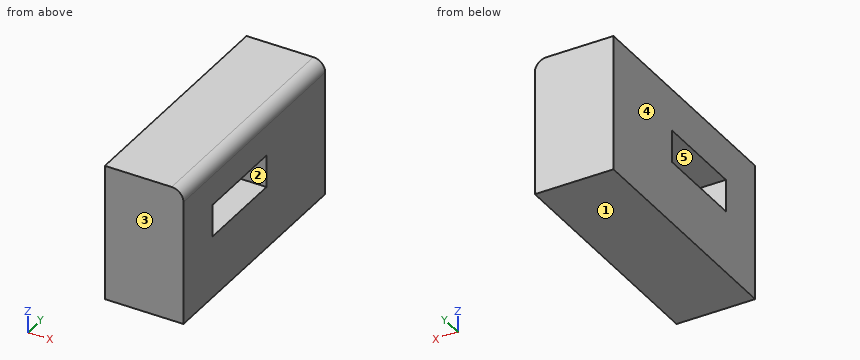
```python
from build123d import *

# Parameters (mm, degrees)
F0_W     = 155.76981
F0_H     = 88.070355
F1_DEPTH = 50.8
F2_R     = 7.62
F3_W     = 59.155117
F3_H     = 20.894366
F4_DEPTH = 50.8


with BuildPart() as f1:
    # F0 (on Right) → F1 (new body)
    with BuildSketch(Plane.YZ):
        with Locations((77.884905, -44.035177)):
            Rectangle(F0_W, F0_H)
    extrude(amount=F1_DEPTH)

    # F2
    f2_edges = [f1.edges().sort_by_distance(p)[0] for p in [
        (50.8, 77.884905, 0),
    ]]
    fillet(f2_edges, radius=F2_R)

    # F3 (on face) → F4 (cut)
    with BuildSketch(Plane.YZ.offset(50.8)):
        with Locations((61.734566, -37.397995)):
            Rectangle(F3_W, F3_H)
    extrude(amount=-F4_DEPTH, mode=Mode.SUBTRACT)


solid = f1.part
```
Model file for the job. Use its own axes, mm. Face numbers are marked on the shaded views. A direction names the side the tool comes from. Coordinates: 2 decimals unless noted, no trailing zeros. Order: outer loops, then holes, each group sorted by start corner. A loop starts at its lowest first (then second) coordinate and runs counter-clockwise, first axis right, second up. Notation, with made-up numbers: M 22.25,24 L 33.25,24 A35 ccw 33.25,57 Z; hole C -14.5,19 d10. An arc over 180 degrees is marked long. Answer as CSV lines item,"result".
(1) Pull direction Z, two halves, no side cores. Call the marked faces 1, 2 and 3: +Z half, -Z half, draft (parallel to the pull), parting line (faces both ways), or undercut.
Geometry says:
face 1,"-Z half"
face 2,"undercut"
face 3,"draft"
(2) Band-saw the part on B-B, the plane x = 38. List the corners of the cut face in (y, z), then the cut area to 3 significant figures.
Geometry says:
outline,"M 0,-88.07 L 155.77,-88.07 L 155.77,0 L 0,0 Z; hole M 32.16,-47.85 L 91.31,-47.85 L 91.31,-26.95 L 32.16,-26.95 Z"
area,"12,500 mm2"
(3) Wall check: line 1 along Z through (x, y) = (42, 87); line 2 along Y through (x, z) = (14, -47); line 3 along Z through (x, y) = (48.5, 68.5). Give the ranges that are in metal, low to high.
Geometry says:
line 1,"z = -88.07 to -47.85, -26.95 to 0"
line 2,"y = 0 to 32.16, 91.31 to 155.77"
line 3,"z = -88.07 to -47.85, -26.95 to -2.16"
(4) Band-saw the part on C-C, the plane y = 36. List the corners of the cut face in (x, z), then the cut area to 3 significant figures.
Geometry says:
outline,"M 0,-88.07 L 50.8,-88.07 L 50.8,-47.85 L 0,-47.85 Z; M 0,-26.95 L 50.8,-26.95 L 50.8,-7.62 A7.62 ccw 43.18,0 L 0,0 Z"
area,"3,400 mm2"
(5) Band-saw the part on A-A, the plane z = -33.5. List the corners of the cut face in (x, y).
Geometry says:
outline,"M 0,0 L 50.8,0 L 50.8,32.16 L 0,32.16 Z; M 0,91.31 L 50.8,91.31 L 50.8,155.77 L 0,155.77 Z"
(6) 3-axis set-ups, long thin cutter, end or side, ignore diameter. For the marked faces 4 and 5: which of +Z, -Z, +X, -X, +Y, -Y reach the whole face in a straight line?
Geometry says:
face 4,"+Z, -Z, -X, +Y, -Y"
face 5,"+X, -X"
